The listing builds one solid part. Answer for the finished solid, in the listing's coordinates (mm). Give positions to 0.01 mm unless a question says otherwise; leave off trailing zeros. Order: outer loops, then holes, each group sorted by start corner. A loop starts at its lowest first (then second) coordinate and runs counter-clockwise, first axis right, second up. Notation, with made-up numbers: (57, -3) - (69, -3) arc R19 ccw to (69, 33) - close; hole circle Ø5 at (22.25, 44). An arc over 180 degrees is marked (long way). Answer in a Markdown table with one row per item.
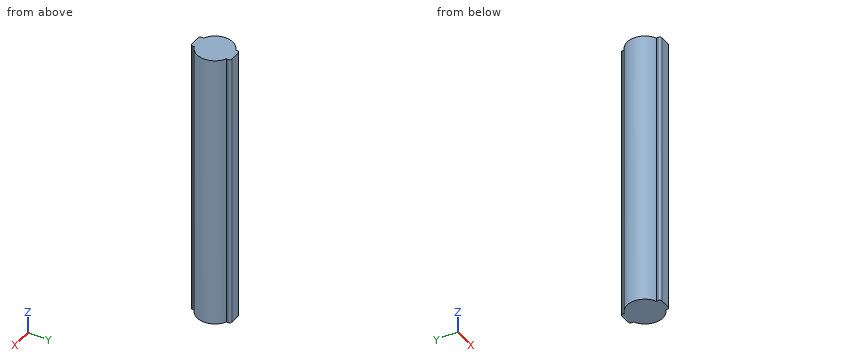
Autodesk Inventor part; units mm, degrees
ref_plane "YZ Plane" through (0, 0, 0) normal (1, 0, 0) x (0, 1, 0)
ref_plane "XZ Plane" through (0, 0, 0) normal (0, 1, 0) x (-1, 0, 0)
ref_plane "XY Plane" through (0, 0, 0) normal (0, 0, 1) x (1, 0, 0)
sketch "Sketch1" plane through (0, 0, 0) normal (0, 0, 1) x (1, 0, 0)
  circle A0 centre (0, 0) radius 3.2
  line L0 (0.9333, -3.6357) -> (-0.9333, -3.6357)
  line L1 (-1.3333, -3.2357) -> (-1.3333, 3.2357)
  line L2 (-0.9333, 3.6357) -> (0.9333, 3.6357)
  line L3 (1.3333, 3.2357) -> (1.3333, -3.2357)
  line L4 (1.3333, -3.6357) -> (-1.3333, 3.6357) construction
  line L5 (-1.3333, -3.6357) -> (1.3333, 3.6357) construction
  arc A1 (-0.9333, 3.6357) -> (-1.3333, 3.2357) centre (-0.9333, 3.2357) ccw
  arc A2 (1.3333, 3.2357) -> (0.9333, 3.6357) centre (0.9333, 3.2357) ccw
  arc A3 (0.9333, -3.6357) -> (1.3333, -3.2357) centre (0.9333, -3.2357) ccw
  arc A4 (-1.3333, -3.2357) -> (-0.9333, -3.6357) centre (-0.9333, -3.2357) ccw
  point P0 (-1.3333, 2.909)
  point P1 (-1.3333, -2.909)
  point P2 (1.3333, -2.909)
  point P3 (1.3333, 2.909)
  point P4 (-0.9416, 2.2076)
  point P5 (-0.9416, -2.2076)
  point P6 (0.9416, -2.2076)
  point P7 (0.9416, 2.2076)
  dimension "d0" = 6.4
  dimension "d1" = 2.6667
  dimension "d2" = 7.2714
  dimension "d3" = 0.4
extrude "Extrusion1" add sketch "Sketch1" along normal blind 50
equation "\"d0\" = D_axel - d_toleransAxel"
equation "\"d3\" = r_filletAxel"
equation "\"d4\" = h_axel"
equation "\"D_axel\" = D_axel_1_2_3"
equation "\"d_axelRing\" = d_axelRing_1_2_3"
equation "\"r_filletAxel\" = r_filletAxel_1_2_3"
equation "\"d_toleransAxel\" = 0.6"
equation "\"h_axel\" = 50"
properties part number "Axel_parametriserad_03"
Item 1: Find section A-A on z = 14. Write down the section's boundary in (x, y), then the cut area to 3 significant figures.
Answer block:
| item | result |
|---|---|
| outline | (-1.33, -3.24) arc R0.4 ccw to (-0.93, -3.64) - (0.93, -3.64) arc R0.4 ccw to (1.33, -3.24) - (1.33, -2.91) arc R3.2 ccw to (1.33, 2.91) - (1.33, 3.24) arc R0.4 ccw to (0.93, 3.64) - (-0.93, 3.64) arc R0.4 ccw to (-1.33, 3.24) - (-1.33, 2.91) arc R3.2 ccw to (-1.33, -2.91) - close |
| area | 34.9 mm² |
Item 2: Find section C-C on y = -0.75. Write down the section's boundary in (x, z), then the cut area to 3 significant figures.
Answer block:
| item | result |
|---|---|
| outline | (-3.11, 0) - (3.11, 0) - (3.11, 50) - (-3.11, 50) - close |
| area | 311 mm² |
Item 3: Find section B-B on x = -2. Write down the section's boundary in (y, z).
Answer block:
| item | result |
|---|---|
| outline | (-2.5, 0) - (2.5, 0) - (2.5, 50) - (-2.5, 50) - close |
Item 4: This flat-tipped pin is pushed along its axis until it touches: P1, Ø1, axis at x = -2.5, z = 15, coming from the -Y side. Where does it stop, or does it pass through?
Answer block:
| item | result |
|---|---|
| P1 | y = -2.5 |
Item 5: Consider line 1 (X direction, y = 0.25, z = 13.5); line 2 (X direction, y = 3, z = 45.5); line 3 (Y direction, x = -2.5, z = 11.5). Determine where each line is inside the solid, lowest interval first.
Answer block:
| item | result |
|---|---|
| line 1 | -3.19 to 3.19 |
| line 2 | -1.33 to 1.33 |
| line 3 | -2 to 2 |
